Job drawing, mm, ordinate dimensions from the low corner. One solid piece. Round coordinates to 2 decimals unless told otherwise and drop trailing zeros. Loops run counter-clockwise (first coordinate to the right, second up) from the corner with the lowest first, then second, coordinate; pieces in that order, holes last.
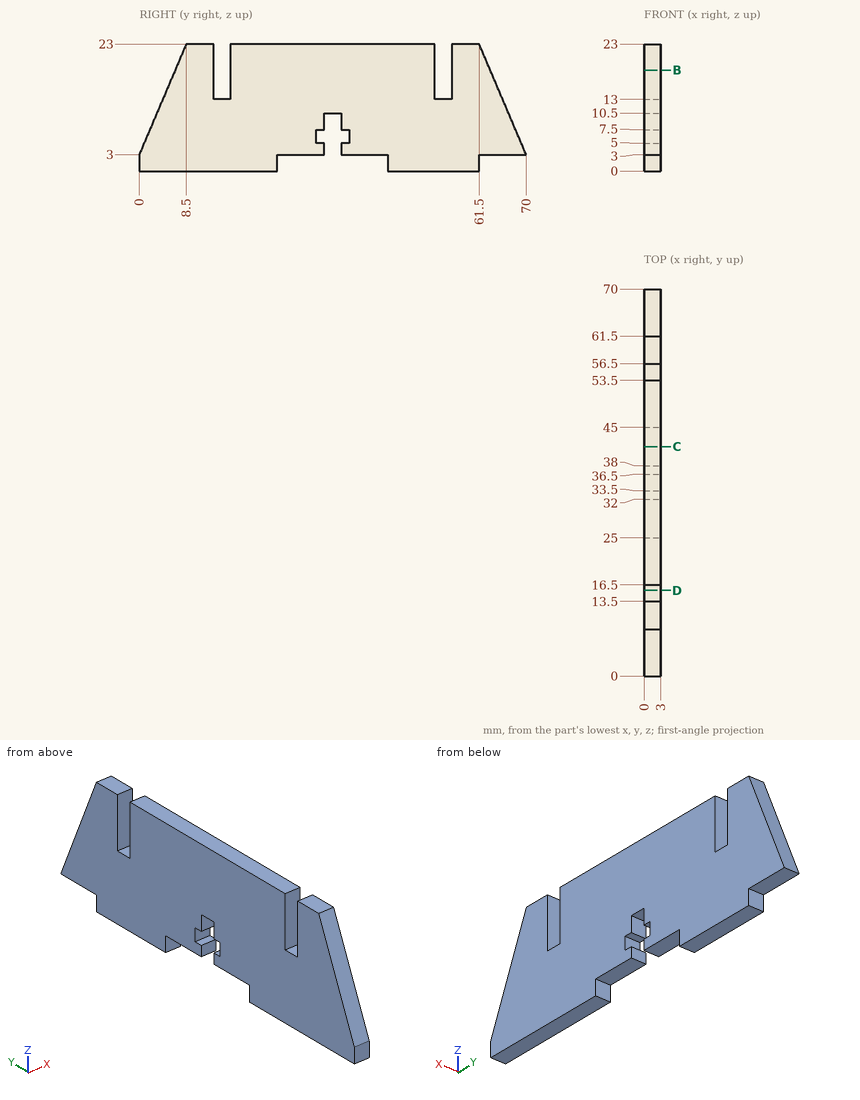
(1) Slice it at C-C on y = 41.5. List the corners of the cut face in (x, z), plus the area to 3 significant figures.
Responses:
outline: (0, 3) - (3, 3) - (3, 23) - (0, 23) - close
area: 60.0 mm2
(2) Slice it at B-B on z = 18.25. List the corners of the cut face in (x, y), plus the area to 3 significant figures.
Responses:
outline: (0, 6.48) - (3, 6.48) - (3, 13.5) - (0, 13.5) - close; (0, 16.5) - (3, 16.5) - (3, 53.5) - (0, 53.5) - close; (0, 56.5) - (3, 56.5) - (3, 63.52) - (0, 63.52) - close
area: 153 mm2
(3) Slice it at D-D on y = 15.5. List the corners of the cut face in (x, z).
Responses:
outline: (0, 0) - (3, 0) - (3, 13) - (0, 13) - close
(4) Pin check, flat tips, straight feed: P1, Ø3, axis at y = 56, z = 9.5, coming from the -X side; P2, Ø0.8, axis at x = 1.5, z = 6.5, coming from the -Y side; P3, Ø0.8, axis at x = 1.5, z = 6.5, coming from the +Y side; P4, Ø1.6, axis at x = 1, y = 33, coming from the -Z side. Stop position of each tip, or through.
Responses:
P1: stops at x = 0
P2: stops at y = 1.32
P3: stops at y = 68.68
P4: stops at z = 3
(5) Probe line 1 (Y direction, x = 1.45, z = 2.25); line 2 (Z direction, x = 1.2, y = 37); line 3 (Y direction, x = 0.9, z = 21.25). List the from-to ranges inside material, lowest first.
Responses:
line 1: y = 0 to 25, 45 to 61.5
line 2: z = 3 to 5, 7.5 to 23
line 3: y = 7.76 to 13.5, 16.5 to 53.5, 56.5 to 62.24
